from build123d import *

# Parameters (mm, degrees)
SKETCH1_R           = 1.6383
SKETCH1_W           = 3.302
SKETCH1_H           = 9.525
BOSS_EXTRUDE1_DEPTH = 3.175


with BuildPart() as part:
    # Sketch1 → Boss-Extrude1 (new body)
    with BuildSketch(Plane.XY):
        with BuildLine():
            Line((-1.5875, 19.685), (1.5875, 19.685))
            ThreePointArc((1.5875, 19.685), (3.83256403, 18.75506403), (4.7625, 16.51))
            Line((4.7625, 16.51), (4.7625, 6.985))
            Line((4.7625, 6.985), (7.9375, 6.985))
            Line((7.9375, 6.985), (7.9375, -0.635))
            ThreePointArc((7.9375, -0.635), (6.077628061, -5.125128061), (1.5875, -6.985))
            Line((1.5875, -6.985), (-1.5875, -6.985))
            ThreePointArc((-1.5875, -6.985), (-6.077628061, -5.125128061), (-7.9375, -0.635))
            Line((-7.9375, -0.635), (-7.9375, 6.985))
            Line((-7.9375, 6.985), (-4.7625, 6.985))
            Line((-4.7625, 6.985), (-4.7625, 16.51))
            ThreePointArc((-4.7625, 16.51), (-3.83256403, 18.75506403), (-1.5875, 19.685))
        make_face()
        with Locations((0, 0.254)):
            Circle(SKETCH1_R, mode=Mode.SUBTRACT)
        with Locations((0, 11.7475)):
            Rectangle(SKETCH1_W, SKETCH1_H, mode=Mode.SUBTRACT)
    extrude(amount=BOSS_EXTRUDE1_DEPTH)


solid = part.part
The listing builds one solid part. Answer for the finished solid, in the listing's coordinates (mm). A direction names the side the tool comes from. Coordinates: 2 decimals unless noted, no trailing zeros. Write each loop counter-clockwise with the first axis right and the second up, starting at its lowest first coordinate (ties: lowest second). Pieces come first, ordered by that corner, then holes. Notation, with made-up numbers: (44.5, 89.25) -> (53.5, 89.25) arc R28 cw to (53.5, 113.25) -> close; hole circle Ø2 at (7, 84.25). An arc over 180 degrees is marked (long way). One line per question, with ' | ' between items.
1. Section A-A (x = 0) is taken. Determine the outline of the cut face in (y, z) (3 decimals).
Verdict:
outline: (-6.985, 0) -> (-1.384, 0) -> (-1.384, 3.175) -> (-6.985, 3.175) -> close; (1.892, 0) -> (6.985, 0) -> (6.985, 3.175) -> (1.892, 3.175) -> close; (16.51, 0) -> (19.685, 0) -> (19.685, 3.175) -> (16.51, 3.175) -> close
2. Section D-D (x = -6.5) is taken. Determine the outline of the cut face in (y, z) (3 decimals), and give its area (3 significant figures).
Verdict:
outline: (-4.659, 0) -> (6.985, 0) -> (6.985, 3.175) -> (-4.659, 3.175) -> close | area: 37.0 mm^2
3. Which of the six approach directions +Z, -Z, +X, -X, +Y, -Y give full straight-line access (tool end or side, diameter ignored) to faces 1 (the flat face through (0, 4, 0)), 2 (the flat face through (6, 6.985, 2)), 3 (the flat face through (0, 16.51, 2)), 4 (the flat face through (-6, 6.985, 2))?
Verdict:
face 1: -Z, +X, -X, +Y, -Y | face 2: +Z, -Z, +X, +Y | face 3: +Z, -Z | face 4: +Z, -Z, -X, +Y
4. Given pin 1 Ø1 at (x, z) = (6.5, 2.5) entering from +Y (3 decimals); pin 2 Ø1 at (y, z) = (12.5, 1) entering from +X, each flat-ended and moving along its own axis, determine where each tip first touches the part or whether it passes through.
Verdict:
pin 1: stops at y = 6.985 | pin 2: stops at x = 4.76
5. Section B-B (z = 1.45) is taken. State how many separate pieces and enclosed holes the cut face has, and give its area (3 significant figures).
Verdict:
separate pieces: 1 | enclosed holes: 2 | area: 281 mm^2
6. For a pull along X with two mould halves and no side action, classify faces 5 (the flat face through (0, -6.985, 2)), 6 (the flat face through (7.938, 3, 2)), 7 (the flat face through (-4.762, 12, 2)), 8 (the cylindrical face through (-1.3, -0.74, 1.57)) as released by +X, released by -X, zero draft, split by the parting line, or undercut.
Verdict:
face 5: zero draft | face 6: released by +X | face 7: released by -X | face 8: undercut
7. Section C-C (x = 6) is taken. Determine the outline of the cut face in (y, z) (3 decimals), and give its area (3 significant figures).
Verdict:
outline: (-5.201, 0) -> (6.985, 0) -> (6.985, 3.175) -> (-5.201, 3.175) -> close | area: 38.7 mm^2
8. Straight lines are drawn through the part: line 1 (Y direction, x = 0, z = 1.85) (3 decimals); line 2 (X direction, y = 16.25, z = 0.8); line 3 (Y direction, x = 0.5, z = 1.05) (3 decimals). For each, find the intervals that lie inside material, in ascending order.
Verdict:
line 1: y = -6.985 to -1.384, 1.892 to 6.985, 16.51 to 19.685 | line 2: x = -4.76 to -1.65, 1.65 to 4.76 | line 3: y = -6.985 to -1.306, 1.814 to 6.985, 16.51 to 19.685
